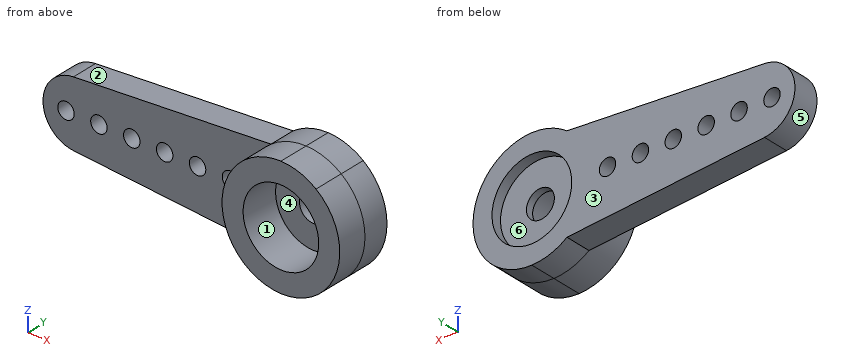
```python
from build123d import *
from build123d.topology import SkipClean

# Parameters (mm, degrees)
SALIENTE_EXTRUIR1_DEPTH       = 1.6
CROQUIS2_R                    = 3.58
SALIENTE_EXTRUIR2_DEPTH       = 1.83
DI_METRO_DE_TALADRO_1_0_1_1_D = 1
CORTAR_EXTRUIR1_DEPTH         = 25.109029429


with BuildPart() as part:
    # Croquis1 → Saliente-Extruir1 (new body)
    with BuildSketch(Plane(origin=(0, 14.27, 0), x_dir=(1, 0, 0), z_dir=(0, 1, 0))):
        with BuildLine():
            Line((8.033254556, 3.025), (20.046175024, 3.905348937))
            ThreePointArc((20.046175024, 3.905348937), (21.9, 5.9), (20.046175024, 7.894651063))
            Line((20.046175024, 7.894651063), (8.033254556, 8.775))
            ThreePointArc((8.033254556, 8.775), (5.9, 9.48), (3.766745444, 8.775))
            Line((3.766745444, 8.775), (-8.246175024, 7.894651063))
            ThreePointArc((-8.246175024, 7.894651063), (-10.1, 5.9), (-8.246175024, 3.905348937))
            Line((-8.246175024, 3.905348937), (3.766745444, 3.025))
            ThreePointArc((3.766745444, 3.025), (5.9, 2.32), (8.033254556, 3.025))
        make_face()
    extrude(amount=-SALIENTE_EXTRUIR1_DEPTH)

    # Croquis2 → Saliente-Extruir2 (add)
    with BuildSketch(Plane.XZ.offset(-12.67)):
        with Locations(Location((5.9, -5.9, 0), (0, 0, 53.424526421))):
            Circle(CROQUIS2_R)
    extrude(amount=SALIENTE_EXTRUIR2_DEPTH)

    # Croquis3 → Cortar-Revoluci_n1 (revolve, cut)
    with BuildSketch(Plane.XY.offset(-5.9), mode=Mode.PRIVATE) as cortar_revoluci_n1_sk:
        Polygon((8.325, 14.27), (5.9, 14.27), (5.9, 10.84), (8.2, 10.84), (8.2, 13.2), (6.75, 13.2), (6.75, 13.65), (8.325, 13.65), align=None)
    revolve(cortar_revoluci_n1_sk.sketch.rotate(Axis((5.9, 14.27, -5.9), (0, -1, 0)), 270), axis=Axis((5.9, 14.27, -5.9), (0, -1, 0)), mode=Mode.SUBTRACT)

    # Di_metro de taladro _1.0 _1_1 (through all)
    with Locations(Plane(origin=(0, 12.67, 0), x_dir=(-1, 0, 0), z_dir=(0, -1, 0))):
        with Locations((2.7, 5.9), (6.7, 5.9), (8.7, 5.9), (4.7, 5.9), (0.7, 5.9), (-10.5, 5.9), (-14.5, 5.9), (-18.5, 5.9), (-20.5, 5.9), (-16.5, 5.9), (-12.5, 5.9), (-1.3, 5.9)):
            Hole(DI_METRO_DE_TALADRO_1_0_1_1_D / 2)

    # Croquis6 → Cortar-Extruir1 (cut, through all)
    with SkipClean():  # the faces are left unmerged after this step: merging them gives an invalid solid
        with BuildSketch(Plane.XZ.offset(-10.84)):
            with BuildLine():
                Line((5.9, -9.48), (5.9, -13.293160377))
                Line((5.9, -13.293160377), (27.115989236, -13.293160377))
                Line((27.115989236, -13.293160377), (27.115989236, 2.204986014))
                Line((27.115989236, 2.204986014), (5.9, 2.204986014))
                Line((5.9, 2.204986014), (5.9, -2.32))
                ThreePointArc((5.9, -2.32), (9.48, -5.9), (5.9, -9.48))
            make_face()
        extrude(amount=-CORTAR_EXTRUIR1_DEPTH, mode=Mode.SUBTRACT)
    add(part.part.scale(1), mode=Mode.REPLACE)  # the faces are merged on a copy


solid = part.part
```
The listing builds one solid part. Answer for the finished solid, in the listing's coordinates (mm). Face numbers are marked on the shaded views. A direction names the side the tool comes from. Give positions to 0.01 mm unless a question says otherwise; leave off trailing zeros. Order: outer loops, then holes, each group sorted by start corner. A loop starts at its lowest first (then second) coordinate and runs counter-clockwise, first axis right, second up.
1) Find section A-A on x = -2.7. Write down the section's boundary in (y, z), then the cut area to 3 significant figures.
Reported:
outline: (12.67, -8.3) - (14.27, -8.3) - (14.27, -6.4) - (12.67, -6.4) - close; (12.67, -5.4) - (14.27, -5.4) - (14.27, -3.5) - (12.67, -3.5) - close
area: 6.08 mm2
2) Find section B-B on z = -5.9. Give the number of separate pieces and of enclosed holes in the cut face, then the cut area to 3 significant figures.
Reported:
separate pieces: 8
enclosed holes: 0
area: 20.2 mm2
3) Find section D-D on x = -8.7. Write down the section's boundary in (y, z), then the cut area to 3 significant figures.
Reported:
outline: (12.67, -7.81) - (14.27, -7.81) - (14.27, -6.4) - (12.67, -6.4) - close; (12.67, -5.4) - (14.27, -5.4) - (14.27, -3.99) - (12.67, -3.99) - close
area: 4.51 mm2
4) For the marked faces 4, 5 and 6, determine the directions among +Z, -Z, +X, -X, +Y, -Y from which every point of the face is accessible in a straight line to the end or side of a thin tool.
Reported:
face 4: -Y
face 5: -X, +Y, -Y
face 6: +Y
5) Consider line 1 along Y through (x, z) = (-4.25, -6.75); line 2 along Y through (x, z) = (4.25, -6.25); line 3 along Z through (x, y) = (-0.7, 13.8). Determine where each line is inside the solid, lowest interval first.
Reported:
line 1: y = 12.67 to 14.27
line 2: y = 13.2 to 13.65
line 3: z = -8.45 to -6.4, -5.4 to -3.35
6) Determine the mould class of the marked faces 1, 2 and 3 for opening direction Z: pulls with the +Z half, pulls with the -Z half, needs draft (parallel to the pull), parting line crosses it, or undercut.
Reported:
face 1: undercut
face 2: pulls with the +Z half
face 3: needs draft
7) Find section C-C on z = -7.5. Write down the section's boundary in (x, y).
Reported:
outline: (-9.3, 12.67) - (2.7, 12.67) - (2.7, 10.84) - (4.25, 10.84) - (4.25, 13.2) - (7.55, 13.2) - (7.55, 10.84) - (9.1, 10.84) - (9.1, 14.27) - (7.72, 14.27) - (7.72, 13.65) - (4.08, 13.65) - (4.08, 14.27) - (-9.3, 14.27) - close
8) Given P1, Ø1.4, axis at x = 6.5, z = -5.5, coming from the -Y side; P2, Ø1, axis at y = 12, z = -6.5, coming from the -X side; P3, Ø4, axis at x = 5.5, z = -7, coming from the +Y side; P4, Ø3, axis at x = -1.5, z = -7, coming from the -Y side, each flat-ended and moving along its own axis, determine where each tip first touches the part or whether it passes through.
Reported:
P1: stops at y = 13.2
P2: stops at x = 2.32
P3: stops at y = 14.27
P4: stops at y = 12.67
